from build123d import *

# Parameters (mm, degrees)
SKETCH_1_W               = 80
SKETCH_1_H               = 80
EXTRUDE_1_DEPTH          = 10.5
SKETCH_3_R               = 1.65
SKETCH_3_R_2             = 10.35
CUT_EXTRUDE_1_DEPTH      = 62.116691664
FILLET_3_R               = 8
FILLET_4_R               = 8
FILLET_5_R               = 8
FILLET_6_R               = 8
EXTRUDE_START            = 6.2
EXTRUDE_2_DEPTH          = 6.2
CUT_EXTRUDE_2_DEPTH      = 62.116691664
CUT_EXTRUDE_2_DEPTH_BACK = 62.116691664
SKETCH_12_R              = 1.65


with BuildPart() as part:
    # 草图1 → 凸台-拉伸1 (new body)
    with BuildSketch(Plane.XY):
        with Locations((-5, 0)):
            Rectangle(SKETCH_1_W, SKETCH_1_H)
    extrude(amount=EXTRUDE_1_DEPTH)

    # 草图3 → 切除-拉伸1 (cut, through all)
    with BuildSketch(Plane.XY.offset(10.5)):
        with Locations((-19.95, 15)):
            Circle(SKETCH_3_R)
        with Locations((-9.86238383, 35)):
            Circle(SKETCH_3_R)
        with Locations((0.16238383, 35)):
            Circle(SKETCH_3_R)
        with Locations((10.25, 15)):
            Circle(SKETCH_3_R_2)
    extrude(amount=-CUT_EXTRUDE_1_DEPTH, mode=Mode.SUBTRACT)

    # 圆角3
    fillet_3_edges = [part.edges().sort_by_distance(p)[0] for p in [
        (35, 40, 5.25),
    ]]
    fillet(fillet_3_edges, radius=FILLET_3_R)

    # 圆角4
    fillet_4_edges = [part.edges().sort_by_distance(p)[0] for p in [
        (-45, 40, 5.25),
    ]]
    fillet(fillet_4_edges, radius=FILLET_4_R)

    # 圆角5
    fillet_5_edges = [part.edges().sort_by_distance(p)[0] for p in [
        (-45, -40, 5.25),
    ]]
    fillet(fillet_5_edges, radius=FILLET_5_R)

    # 圆角6
    fillet_6_edges = [part.edges().sort_by_distance(p)[0] for p in [
        (35, -40, 5.25),
    ]]
    fillet(fillet_6_edges, radius=FILLET_6_R)

    # 草图11 → 凸台-拉伸2 (add)
    with BuildSketch(Plane.XY.offset(10.5).offset(EXTRUDE_START)):
        with BuildLine():
            Line((-45, 0), (-37, 0))
            Line((-37, 0), (-37, -32))
            Line((-37, -32), (27, -32))
            Line((27, -32), (27, 0))
            Line((27, 0), (35, 0))
            Line((35, 0), (35, -32))
            ThreePointArc((35, -32), (32.656854249, -37.656854249), (27, -40))
            Line((27, -40), (-37, -40))
            ThreePointArc((-37, -40), (-42.656854249, -37.656854249), (-45, -32))
            Line((-45, -32), (-45, 0))
        make_face()
    extrude(amount=-EXTRUDE_2_DEPTH)

    # 草图12 → 切除-拉伸2 (cut, two sides: drawn at the far end of the back side and taken through both)
    with BuildSketch(Plane.XY.offset(10.5).offset(-CUT_EXTRUDE_2_DEPTH_BACK)):
        with Locations((29.828427125, -34.828427125)):
            Circle(SKETCH_12_R)
        with Locations((-39.828427125, -34.828427125)):
            Circle(SKETCH_12_R)
        with Locations((-39.828427125, -5)):
            Circle(SKETCH_12_R)
        with Locations((29.828427125, -5)):
            Circle(SKETCH_12_R)
    extrude(amount=CUT_EXTRUDE_2_DEPTH + CUT_EXTRUDE_2_DEPTH_BACK, mode=Mode.SUBTRACT)


solid = part.part
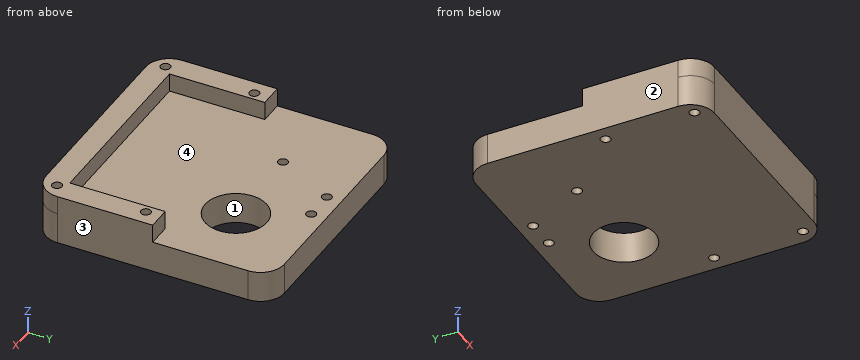
Check sheet for the modelled part. Datum: model origin and axes. Units: mm. Face numbers are marked on the shaded views. Round coordinates to 2 decimals unless told otherwise and drop trailing zeros. Loops run counter-clockwise (first coordinate to the right, second up) from the corner with the lowest first, then second, coordinate; pieces in that order, holes last. Notation, with made-up numbers: M 8.25,-18.5 L 32.25,-18.5 A23 ccw 32.25,0.5 Z; hole C 70.25,55.5 d8. An arc over 180 degrees is marked long. One line per question, with ' | ' between items. Start each with the question number.
Item 1: Section check A-A (x = -19.95). Record the boundary of the cut face in (y, z).
Item 2: Section check C-C (z = 14.5). Record the boundary of the cut face in (x, y).
Item 3: Gauge pin test, flat ends, axial feed: pin 1 Ø24 at (x, y) = (10.25, 15) entering from -Z; pin 2 Ø1.9 at (x, z) = (31.5, 14) entering from +Y; pin 3 Ø3 at (x, y) = (-20, -19.5) entering from +Z; pin 4 Ø2 at (x, y) = (0.16, 35) entering from +Z. Record the tip position at first contact, or that the pin passes through.
Item 4: Section check D-D (y = 8.5). Record the boundary of the cut face in (x, z).
Item 5: Scan lines: probe 1 along X at (y, z) = (-5, 9.25); probe 2 along X at (y, z) = (-5, 13); probe 3 along X at (y, z) = (-10, 13). Record each from-to range of solid material in increasing order.
Item 6: Release check for a two-part mould opening along X. For the marked faces 1, 2, 3 and 4 record: released by +X, released by -X, zero draft, split by the parting line, or undercut.
Item 7: Section check B-B (y = -5). Record the boundary of the cut face in (x, z), and give its area (3 significant figures).
Worked out:
1) outline: M -40,0 L 13.35,0 L 13.35,10.5 L -32,10.5 L -32,16.7 L -40,16.7 Z; M 16.65,0 L 40,0 L 40,10.5 L 16.65,10.5 Z
2) outline: M -45,-32 A8 ccw -37,-40 L 27,-40 A8 ccw 35,-32 L 35,0 L 27,0 L 27,-32 L -37,-32 L -37,0 L -45,0 Z; hole C -39.83,-34.83 d3.3; hole C -39.83,-5 d3.3; hole C 29.83,-34.83 d3.3; hole C 29.83,-5 d3.3
3) pin 1: z = 0 | pin 2: y = 0 | pin 3: z = 10.5 | pin 4: through
4) outline: M -45,0 L 2.2,0 L 2.2,10.5 L -45,10.5 Z; M 18.3,0 L 35,0 L 35,10.5 L 18.3,10.5 Z
5) probe 1: -45 to -41.48, -38.18 to 28.18, 31.48 to 35 | probe 2: -45 to -41.48, -38.18 to -37, 27 to 28.18, 31.48 to 35 | probe 3: -45 to -37, 27 to 35
6) face 1: undercut | face 2: released by -X | face 3: released by +X | face 4: undercut
7) outline: M -45,0 L -41.48,0 L -41.48,16.7 L -45,16.7 Z; M -38.18,0 L 28.18,0 L 28.18,16.7 L 27,16.7 L 27,10.5 L -37,10.5 L -37,16.7 L -38.18,16.7 Z; M 31.48,0 L 35,0 L 35,16.7 L 31.48,16.7 Z | area: 829 mm^2
